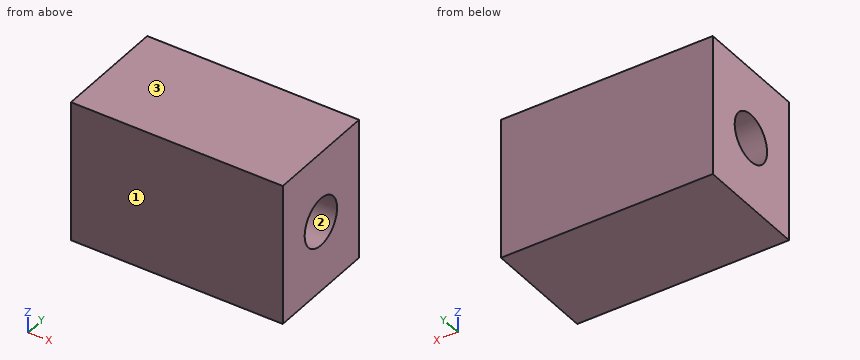
```python
from build123d import *

# Parameters (mm, degrees)
SKETCH2_W               = 30
SKETCH2_H               = 20
BOSS_EXTRUDE1_DEPTH     = 8
CUT_EXTRUDE1_DEPTH      = 20.723082923
CUT_EXTRUDE1_DEPTH_BACK = 20.723082923
SKETCH5_R               = 3.4


with BuildPart() as part:
    # Sketch2 → Boss-Extrude1 (new, symmetric)
    with BuildSketch(Plane(origin=(0, 0, 0), x_dir=(1, 0, 0), z_dir=(0, 1, 0))):
        Rectangle(SKETCH2_W, SKETCH2_H)
    extrude(amount=BOSS_EXTRUDE1_DEPTH, both=True)

    # Sketch5 → Cut-Extrude1 (cut, two sides: drawn at the far end of the back side and taken through both)
    with BuildSketch(Plane(origin=(0, 0, 0), x_dir=(0, 0, -1), z_dir=(1, 0, 0)).offset(-CUT_EXTRUDE1_DEPTH_BACK)):
        Circle(SKETCH5_R)
    extrude(amount=CUT_EXTRUDE1_DEPTH + CUT_EXTRUDE1_DEPTH_BACK, mode=Mode.SUBTRACT)


solid = part.part
```
The model under review builds one solid part; all positions refer to its coordinate system, in mm. Face numbers are marked on the shaded views. Give positions to 0.01 mm unless a question says otherwise; leave off trailing zeros. Write each loop counter-clockwise with the first axis right and the second up, starting at its lowest first coordinate (ties: lowest second). Pieces come first, ordered by that corner, then holes. Notation, with made-up numbers: (28, -8) - (40, -8) arc R22 ccw to (40, 11) - close; hole circle Ø3 at (81.25, -29). An arc over 180 degrees is marked (long way). Answer in a Markdown table with one row per item. Add a question column.
1. Draft analysis for pull direction Y (two halves, no side actions). For the marked faces 1, 2 and 3, state which applies: +Y half, -Y half, draft (parallel to the pull), parting line (faces both ways), or undercut.
2. We need section A-A on z = 0. Write out the cut boundary in (x, y).
3. We need section C-C on x = 6.75. Write out the cut boundary in (y, z), then the cut area to 3 significant figures.
4. Wall thickness on line 1 along Y through (x, z) = (-7, 0); line 2 along Z through (x, y) = (-6.5, 0); line 3 along Z through (x, y) = (0.5, 1.25): over which ranges is each line inside the solid? List them lowest first. Write a range as [from, to].
5. We need section B-B on y = 0. Write out the cut boundary in (x, z), then the cut area to 3 significant figures.
Ans:
| question | item | result |
|---|---|---|
| 1 | face 1 | -Y half |
| 1 | face 2 | undercut |
| 1 | face 3 | draft |
| 2 | outline | (-15, -8) - (15, -8) - (15, -3.4) - (-15, -3.4) - close; (-15, 3.4) - (15, 3.4) - (15, 8) - (-15, 8) - close |
| 3 | outline | (-8, -10) - (8, -10) - (8, 10) - (-8, 10) - close; hole circle Ø6.8 at (0, 0) |
| 3 | area | 284 mm^2 |
| 4 | line 1 | y = [-8, -3.4], [3.4, 8] |
| 4 | line 2 | z = [-10, -3.4], [3.4, 10] |
| 4 | line 3 | z = [-10, -3.16], [3.16, 10] |
| 5 | outline | (-15, -10) - (15, -10) - (15, -3.4) - (-15, -3.4) - close; (-15, 3.4) - (15, 3.4) - (15, 10) - (-15, 10) - close |
| 5 | area | 396 mm^2 |
